Check sheet for the drawn part. Datum: minimum x, y, z corner. Units: mm. A direction names the side the tool comes from. Give positions to 0.01 mm unless a question says otherwise; leave off trailing zeros. Order: outer loops, then holes, each group sorted by start corner. A loop starts at its lowest first (then second) coordinate and runs counter-clockwise, first axis right, second up.
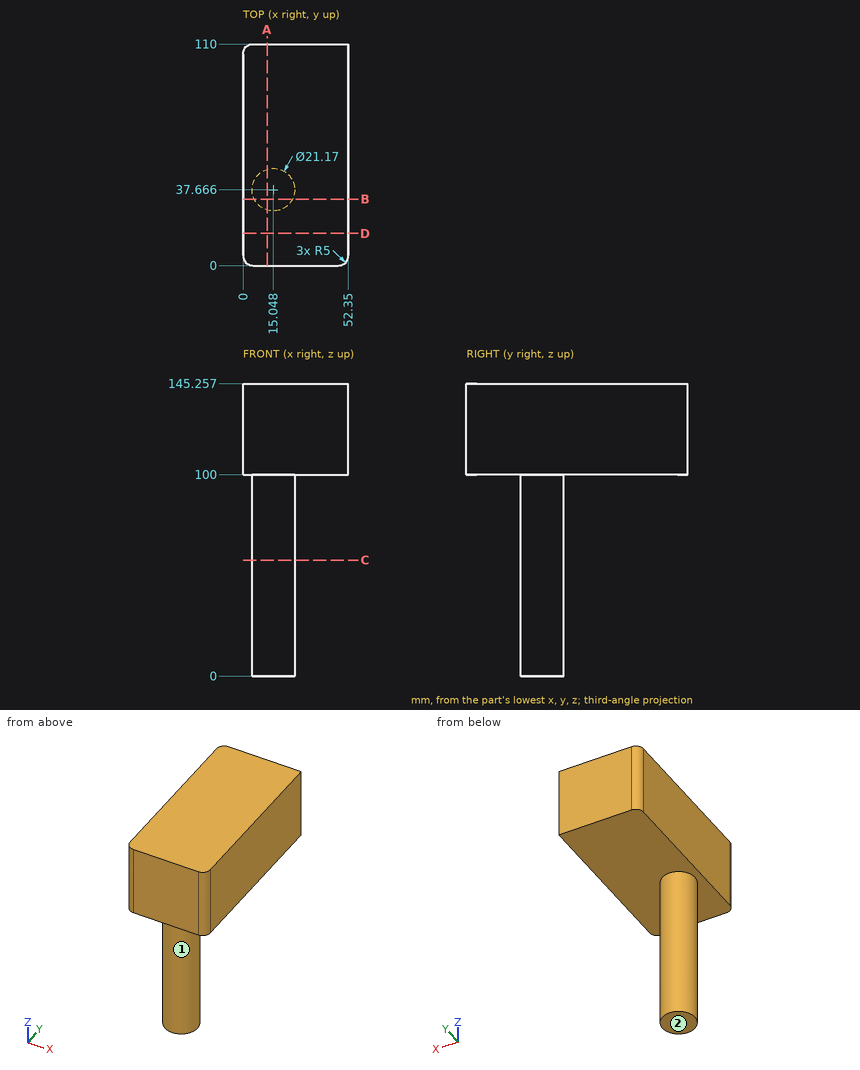
(1) Go/stop test with a flat-tipped pin: pin 1 (4 mm diameter, centred on y = 40, z = 55, fed in from +X). Record where the tip stops, or that it passes through.
Solved:
pin 1: stops at x = 25.63
(2) Scan lines: line 1 (Z direction, x = 3, y = 40.5); line 2 (X direction, y = 32, z = 13); line 3 (Y direction, x = 18, z = 35). Record each from-to range of solid material in increasing order.
Solved:
line 1: z = 100 to 145.26
line 2: x = 6.11 to 23.99
line 3: y = 27.5 to 47.83
(3) Set-up check for the marked faces 1 and 2: record each of +Z, -Z, +X, -X, +Y, -Y from which the full face is reachable in a straight line by a thin tool's end or side.
Solved:
face 1: -Z
face 2: -Z, +X, -X, +Y, -Y
(4) Section check A-A, the plane x = 12. Enter the section's corners in (y, z), then the cut area to 3 significant figures.
Solved:
outline: (0, 100) - (27.53, 100) - (27.53, 0) - (47.8, 0) - (47.8, 100) - (110, 100) - (110, 145.26) - (0, 145.26) - close
area: 7,010 mm2
(5) Section check B-B, the plane y = 33. Enter the section's corners in (x, z).
Solved:
outline: (0, 100) - (5.55, 100) - (5.55, 0) - (24.55, 0) - (24.55, 100) - (52.35, 100) - (52.35, 145.26) - (0, 145.26) - close
(6) Section check C-C, the plane z = 57.5. Enter the section's corners in (x, y) (1 decimal), then the cut area to 3 significant figures.
Solved:
outline: circle Ø21.2 at (15, 37.7)
area: 352 mm2
(7) Section check D-D, the plane y = 16. Enter the section's corners in (x, z).
Solved:
outline: (0, 100) - (52.35, 100) - (52.35, 145.26) - (0, 145.26) - close
